Can you work these out from the model? Positions are in its coordinate system, mm. Give positions to 0.01 mm unless a question says otherwise; leave off trailing zeros. Loops run counter-clockwise (first coordinate to the right, second up) from the corner with the lowest first, then second, coordinate; pieces in that order, holes last. Notation, with made-up numbers: (87, 69.5) - (115, 69.5) arc R27 cw to (115, 102.5) - close; hole circle Ø4 at (-13, -13.75). An arc over 180 degrees is marked (long way). Answer in a Markdown table with one row per item.
from build123d import *

# Parameters (mm, degrees)
SKETCH1_W           = 10
SKETCH1_H           = 25
BOSS_EXTRUDE1_DEPTH = 1
CHAMFER1_SIZE       = 0.8
CHAMFER1_SIZE2      = 9.943064816


with BuildPart() as part:
    # Sketch1 → Boss-Extrude1 (new body)
    with BuildSketch(Plane.XY):
        with Locations((-5, 12.5)):
            Rectangle(SKETCH1_W, SKETCH1_H)
    extrude(amount=BOSS_EXTRUDE1_DEPTH)

    # Chamfer1
    chamfer1_edges = [part.edges().sort_by_distance(p)[0] for p in [
        (0, 12.5, 1),
    ]]
    chamfer1_side = [part.faces().sort_by_distance(p)[0] for p in [
        (0, 12.5, 0.5),
    ]]
    chamfer(chamfer1_edges, length=CHAMFER1_SIZE, length2=CHAMFER1_SIZE2, reference=chamfer1_side[0])


solid = part.part
Q1. Imagine slicing it at A-A, the plane y = 4.25. Write out the boundary of the cut face in (x, z).
Checked values:
| item | result |
|---|---|
| outline | (-10, 0) - (0, 0) - (0, 0.2) - (-9.94, 1) - (-10, 1) - close |
Q2. For pin 1 (4 mm diameter, centred on x = -8.5, y = 16, fed in from +Z), with a flat end and sliding along its axis, tell me the tip position at first contact or that it passes through.
Checked values:
| item | result |
|---|---|
| pin 1 | stops at z = 1 |
Q3. If I drill on line 1 (Z direction, x = -2.5, y = 10.75); line 2 (Z direction, x = -4, y = 15), over which ranges is the centre line in solid material (lowest first)? Write a range as [from, to].
Checked values:
| item | result |
|---|---|
| line 1 | z = [0, 0.4] |
| line 2 | z = [0, 0.52] |
Q4. Imagine slicing it at C-C, the plane z = 0.5. Write out the boundary of the cut face in (x, y), and give its area (3 significant figures).
Checked values:
| item | result |
|---|---|
| outline | (-10, 0) - (-3.73, 0) - (-3.73, 25) - (-10, 25) - close |
| area | 157 mm² |
Q5. Imagine slicing it at B-B, the plane x = -1.25. Write out the boundary of the cut face in (y, z).
Checked values:
| item | result |
|---|---|
| outline | (0, 0) - (25, 0) - (25, 0.3) - (0, 0.3) - close |
